Here's how the part is built. I have some questions about the finished solid (model axes, mm). A direction names the side the tool comes from. Round coordinates to 2 decimals unless told otherwise and drop trailing zeros. Write each loop counter-clockwise with the first axis right and the second up, starting at its lowest first coordinate (ties: lowest second). Pieces come first, ordered by that corner, then holes. Notation, with made-up numbers: (43, 83) -> (66, 83) arc R16 ccw to (66, 99) -> close; hole circle Ø7 at (25, -22.5). An arc over 180 degrees is marked (long way). Answer in a Markdown table with one row per item. Add a question column.
from build123d import *

# Parameters (mm, degrees)
SKETCH1_W                      = 127
SKETCH1_H                      = 25.4
BOSS_EXTRUDE1_DEPTH            = 25.4
SKETCH2_W                      = 22.225
SKETCH2_H                      = 22.225
CUT_EXTRUDE1_DEPTH             = 132.982271537
F_7_0_201_DIAMETER_HOLE1_D     = 5.1054
F_7_0_201_DIAMETER_HOLE1_DEPTH = 25.4
F_7_0_201_DIAMETER_HOLE2_D     = 5.1054


with BuildPart() as part:
    # Sketch1 → Boss-Extrude1 (new body)
    with BuildSketch(Plane(origin=(0, 25.4, 0), x_dir=(1, 0, 0), z_dir=(0, 1, 0))):
        with Locations((63.5, -12.7)):
            Rectangle(SKETCH1_W, SKETCH1_H)
    extrude(amount=-BOSS_EXTRUDE1_DEPTH)

    # Sketch2 → Cut-Extrude1 (cut, through all)
    with BuildSketch(Plane(origin=(127, 0, 0), x_dir=(0, 0, -1), z_dir=(1, 0, 0))):
        with Locations((-14.2875, 14.2875)):
            Rectangle(SKETCH2_W, SKETCH2_H)
    extrude(amount=-CUT_EXTRUDE1_DEPTH, mode=Mode.SUBTRACT)

    # #7 (0.201) Diameter Hole1
    with Locations(Plane.XZ):
        with Locations((-12.7, -12.7), (38.1, 12.7), (63.5, 12.7), (88.9, 12.7), (114.3, 12.7)):
            Hole(F_7_0_201_DIAMETER_HOLE1_D / 2, depth=F_7_0_201_DIAMETER_HOLE1_DEPTH)

    # #7 (0.201) Diameter Hole2 (through all)
    with Locations(Plane.XY.offset(3.175)):
        with Locations((12.7, 12.7), (38.1, 12.7), (63.5, 12.7), (88.9, 12.7), (114.3, 12.7)):
            Hole(F_7_0_201_DIAMETER_HOLE2_D / 2)


solid = part.part
Item 1: If we section it at D-D on z = 12.7: Please give me the cut outline in (x, y) (3 decimals).
Item 2: If we mould it in two halves opening along Z, with no side actions, what happens to faces 3 (the cylindrical face through (66.05, 1.61, 12.81)), 4 (the flat face through (63, 2, 25.4)), 5 (the flat face through (63, 25.4, 2))? For each: pulls with the +Z half, pulls with the -Z half, needs draft (parallel to the pull), parting line crosses it, or undercut.
Item 3: If we section it at B-B on y = 12.7: Please give me the cut outline in (x, z) (3 decimals).
Item 4: If we section it at A-A on x = 114.3: Please give me the cut outline in (y, z) (3 decimals).
Item 5: On a 3-axis mill with a long thin cutter (end or side, diameter ignored), from which of +Z, -Z, +X, -X, +Y, -Y can I reach the whole of each face in a straight line? I mean faces 1 (the flat face through (64, 17, 3.175)), 2 (the flat face through (0, 2, 7)). Say none if no direction works.
Item 6: If we section it at C-C on x = 12.7: Please give me the cut outline in (y, z) (3 decimals).
Item 7: For P1, Ø6, axis at x = 88.9, y = 12.7, coming from the -Z side; P2, Ø3, axis at x = 17, y = 15, coming from the +Z side (3 decimals), each with a flat end and sliding along its axis, tell me the tip position at first contact or that it passes through.
Item 8: I need wall thicknesses on line 1 along X through (y, z) = (1.5, 12.5); line 2 along Y through (x, z) = (12.7, 1.65). Which ranges of each line are inside material? Lowest first, please. Write a range as from..to.
Results list:
| question | item | result |
|---|---|---|
| 1 | outline | (0, 0) -> (35.547, 0) -> (35.547, 3.175) -> (0, 3.175) -> close; (40.653, 0) -> (60.947, 0) -> (60.947, 3.175) -> (40.653, 3.175) -> close; (66.053, 0) -> (86.347, 0) -> (86.347, 3.175) -> (66.053, 3.175) -> close; (91.453, 0) -> (111.747, 0) -> (111.747, 3.175) -> (91.453, 3.175) -> close; (116.853, 0) -> (127, 0) -> (127, 3.175) -> (116.853, 3.175) -> close |
| 2 | face 3 | undercut |
| 2 | face 4 | pulls with the +Z half |
| 2 | face 5 | needs draft |
| 3 | outline | (0, 0) -> (10.147, 0) -> (10.147, 3.175) -> (0, 3.175) -> close; (15.253, 0) -> (35.547, 0) -> (35.547, 3.175) -> (15.253, 3.175) -> close; (40.653, 0) -> (60.947, 0) -> (60.947, 3.175) -> (40.653, 3.175) -> close; (66.053, 0) -> (86.347, 0) -> (86.347, 3.175) -> (66.053, 3.175) -> close; (91.453, 0) -> (111.747, 0) -> (111.747, 3.175) -> (91.453, 3.175) -> close; (116.853, 0) -> (127, 0) -> (127, 3.175) -> (116.853, 3.175) -> close |
| 4 | outline | (0, 0) -> (10.147, 0) -> (10.147, 3.175) -> (3.175, 3.175) -> (3.175, 10.147) -> (0, 10.147) -> close; (0, 15.253) -> (3.175, 15.253) -> (3.175, 25.4) -> (0, 25.4) -> close; (15.253, 0) -> (25.4, 0) -> (25.4, 3.175) -> (15.253, 3.175) -> close |
| 5 | face 1 | +Z, +X, -X, +Y |
| 5 | face 2 | +Z, -Z, -X, +Y, -Y |
| 6 | outline | (0, 0) -> (10.147, 0) -> (10.147, 3.175) -> (3.175, 3.175) -> (3.175, 25.4) -> (0, 25.4) -> close; (15.253, 0) -> (25.4, 0) -> (25.4, 3.175) -> (15.253, 3.175) -> close |
| 7 | P1 | z = 0 |
| 7 | P2 | z = 3.175 |
| 8 | line 1 | 0..35.56, 40.64..60.96, 66.04..86.36, 91.44..111.76, 116.84..127 |
| 8 | line 2 | 0..10.15, 15.25..25.4 |
